Can you work these out from the model? Positions are in its coordinate system, mm. Face numbers are marked on the shaded views. Coordinates: 2 decimals unless noted, no trailing zeros. Order: outer loops, then holes, each group sorted by start corner. A loop starts at its lowest first (then second) coordinate and runs counter-clockwise, first axis right, second up. Notation, with made-up numbers: (-9, 6.5) -> (1, 6.5) arc R32 cw to (1, 35.5) -> close; hole circle Ø10 at (15.5, 71.5). An arc over 180 degrees is marked (long way). Use a Markdown table: item, result. Add a question column.
1. We'd pull the mould along Y, two halves only. Please class the marked faces 1, 2, 3 and 4: pulls with the +Y half, pulls with the -Y half, needs draft (parallel to the pull), parting line crosses it, or undercut.
2. If I drill on line 1 along Y through (x, z) = (-146, 16.5); line 2 along Z through (x, y) = (-29.5, 11); line 3 along Y through (x, z) = (-151.5, 14), over which ranges is the centre line in solid material (lowest first)? Write a range as from..to.
3. Suppose I cut it at A-A, the plane z = 16.25. List the corners of the cut face in (x, y) for me.
4. Suppose I cut it at C-C, the plane x = -16. List the corners of the cut face in (y, z) for me.
5. For pin 1 Ø10 at (y, z) = (7, 4) entering from +X; pin 2 Ø1 at (x, y) = (-15, 11) entering from +Z; pin 3 Ø21 at (x, y) = (-146, 0) entering from +Z, each with a flat end and sliding along its axis, tell me the tip position at first contact or that it passes through.
Autodesk Inventor part; units mm, degrees
ref_plane "YZ Plane" through (0, 0, 0) normal (1, 0, 0) x (0, 1, 0)
ref_plane "XZ Plane" through (0, 0, 0) normal (0, 1, 0) x (-1, 0, 0)
ref_plane "XY Plane" through (0, 0, 0) normal (0, 0, 1) x (1, 0, 0)
sketch "Sketch1" plane through (0, 0, 0) normal (0, 0, 1) x (1, 0, 0)
  circle A0 centre (0, 0) radius 25
  circle A1 centre (-146, 0) radius 25
  line L0 (-146, 25) -> (0, 25)
  line L1 (-146, -25) -> (0, -25)
  point P0 (-171, 0)
  point P1 (25, 0)
  dimension "d0" = 50
  dimension "d1" = 196
extrude "Extrusion1" add sketch "Sketch1" along normal blind 20
sketch "Sketch2" plane through (0, 0, 20) normal (0, 0, 1) x (1, 0, 0)
  arc A0 (0, -25) -> (0, 25) centre (0, 0) ccw
  line L0 (0, 25) -> (-146, 25)
  arc A1 (-146, 25) -> (-146, -25) centre (-146, 0) ccw
  line L1 (-146, -25) -> (0, -25)
  circle A2 centre (-146, 0) radius 20
  dimension "d4" = 40
extrude "Extrusion2" add sketch "Sketch2" along normal blind 0.5 contours A2
chamfer "Chamfer1" distance 0.5 angle 45 1 edges at (-166, 0, 20.5)
sketch "Sketch3" plane through (-146, 0, 20.5) normal (0, 0, 1) x (1, 0, 0)
  circle A0 centre (0, 0) radius 20
  arc A1 (146, -25) -> (146, 25) centre (146, 0) ccw
  line L0 (146, 25) -> (0, 25)
  arc A2 (0, 25) -> (0, -25) centre (0, 0) ccw
  line L1 (0, -25) -> (146, -25)
  circle A3 centre (0, 0) radius 13
  dimension "d10" = 26
extrude "Extrusion3" cut sketch "Sketch3" against normal blind 10 contours A3
fillet "Fillet1" radius 2 8 edges at (25, 0, 20) (-73, 25, 20) (-171, 0, 20) (-73, -25, 20) (25, 0, 0) (-73, 25, 0) (-171, 0, 0) (-73, -25, 0)
properties part number "HMI arm bewegende deel" material "Steel"
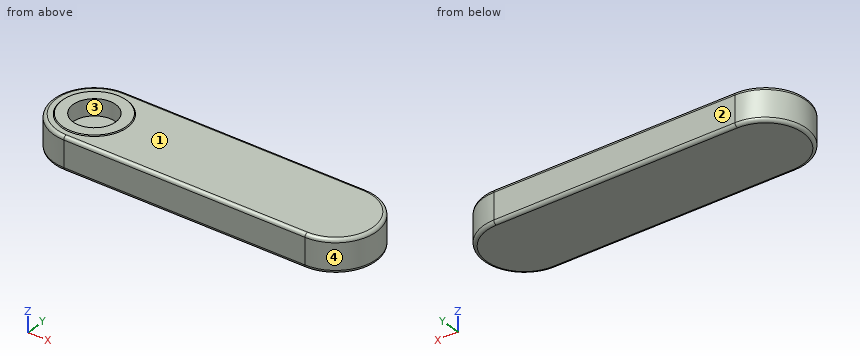
Worked out:
| question | item | result |
|---|---|---|
| 1 | face 1 | needs draft |
| 1 | face 2 | pulls with the +Y half |
| 1 | face 3 | undercut |
| 1 | face 4 | parting line crosses it |
| 2 | line 1 | y = -25..-13, 13..25 |
| 2 | line 2 | z = 0..20 |
| 2 | line 3 | y = -24.39..-11.78, 11.78..24.39 |
| 3 | outline | (-146, -25) -> (0, -25) arc R25 ccw to (0, 25) -> (-146, 25) arc R25 ccw to start; hole circle Ø26 at (-146, 0) |
| 4 | outline | (-25, 2) arc R2 ccw to (-23, 0) -> (23, 0) arc R2 ccw to (25, 2) -> (25, 18) arc R2 ccw to (23, 20) -> (-23, 20) arc R2 ccw to (-25, 18) -> close |
| 5 | pin 1 | stops at x = 24.92 |
| 5 | pin 2 | stops at z = 20 |
| 5 | pin 3 | stops at z = 10.5 |
